from build123d import *

# Parameters (mm, degrees)
CROQUIS1_W              = 991
CROQUIS1_H              = 1639
SALIENTE_EXTRUIR1_DEPTH = 5
CROQUIS2_W              = 971
CROQUIS2_H              = 1619
CORTAR_EXTRUIR1_DEPTH   = 2
CROQUIS3_W              = 991
CROQUIS3_H              = 1639
CROQUIS3_W_2            = 989
CROQUIS3_H_2            = 1637
SALIENTE_EXTRUIR2_DEPTH = 30
CROQUIS4_W              = 991
CROQUIS4_H              = 1639
CROQUIS4_W_2            = 921
CROQUIS4_H_2            = 1569
SALIENTE_EXTRUIR3_DEPTH = 1
CROQUIS5_R              = 2.5
CORTAR_EXTRUIR2_DEPTH   = 1


with BuildPart() as part:
    # Croquis1 → Saliente-Extruir1 (new body)
    with BuildSketch(Plane.XY):
        Rectangle(CROQUIS1_W, CROQUIS1_H)
    extrude(amount=SALIENTE_EXTRUIR1_DEPTH)

    # Croquis2 → Cortar-Extruir1 (cut)
    with BuildSketch(Plane.XY.offset(5)):
        Rectangle(CROQUIS2_W, CROQUIS2_H)
    extrude(amount=-CORTAR_EXTRUIR1_DEPTH, mode=Mode.SUBTRACT)

    # Croquis3 → Saliente-Extruir2 (add)
    with BuildSketch(Plane(origin=(0, 0, 0), x_dir=(-1, 0, 0), z_dir=(0, 0, -1))):
        Rectangle(CROQUIS3_W, CROQUIS3_H)
        Rectangle(CROQUIS3_W_2, CROQUIS3_H_2, mode=Mode.SUBTRACT)
    extrude(amount=SALIENTE_EXTRUIR2_DEPTH)

    # Croquis4 → Saliente-Extruir3 (add)
    with BuildSketch(Plane(origin=(0, 0, -30), x_dir=(-1, 0, 0), z_dir=(0, 0, -1))):
        Rectangle(CROQUIS4_W, CROQUIS4_H)
        Rectangle(CROQUIS4_W_2, CROQUIS4_H_2, mode=Mode.SUBTRACT)
    extrude(amount=-SALIENTE_EXTRUIR3_DEPTH)

    # Croquis5 → Cortar-Extruir2 (cut)
    with BuildSketch(Plane(origin=(0, 0, -30), x_dir=(-1, 0, 0), z_dir=(0, 0, -1))):
        with Locations((-478, 0)):
            Circle(CROQUIS5_R)
        with Locations((478, 0)):
            Circle(CROQUIS5_R)
        with BuildLine():
            Line((-473, 652.5), (-473, 648.5))
            ThreePointArc((-473, 648.5), (-478, 643.5), (-483, 648.5))
            Line((-483, 648.5), (-483, 652.5))
            ThreePointArc((-483, 652.5), (-478, 657.5), (-473, 652.5))
        make_face()
        with BuildLine():
            Line((-473, 398.5), (-473, 402.5))
            ThreePointArc((-473, 402.5), (-478, 407.5), (-483, 402.5))
            Line((-483, 402.5), (-483, 398.5))
            ThreePointArc((-483, 398.5), (-478, 393.5), (-473, 398.5))
        make_face()
        with BuildLine():
            Line((-473, -652.5), (-473, -648.5))
            ThreePointArc((-473, -648.5), (-478, -643.5), (-483, -648.5))
            Line((-483, -648.5), (-483, -652.5))
            ThreePointArc((-483, -652.5), (-478, -657.5), (-473, -652.5))
        make_face()
        with BuildLine():
            Line((-473, -398.5), (-473, -402.5))
            ThreePointArc((-473, -402.5), (-478, -407.5), (-483, -402.5))
            Line((-483, -402.5), (-483, -398.5))
            ThreePointArc((-483, -398.5), (-478, -393.5), (-473, -398.5))
        make_face()
        with BuildLine():
            Line((473, -652.5), (473, -648.5))
            ThreePointArc((473, -648.5), (478, -643.5), (483, -648.5))
            Line((483, -648.5), (483, -652.5))
            ThreePointArc((483, -652.5), (478, -657.5), (473, -652.5))
        make_face()
        with BuildLine():
            Line((473, -398.5), (473, -402.5))
            ThreePointArc((473, -402.5), (478, -407.5), (483, -402.5))
            Line((483, -402.5), (483, -398.5))
            ThreePointArc((483, -398.5), (478, -393.5), (473, -398.5))
        make_face()
        with BuildLine():
            Line((473, 398.5), (473, 402.5))
            ThreePointArc((473, 402.5), (478, 407.5), (483, 402.5))
            Line((483, 402.5), (483, 398.5))
            ThreePointArc((483, 398.5), (478, 393.5), (473, 398.5))
        make_face()
        with BuildLine():
            Line((473, 652.5), (473, 648.5))
            ThreePointArc((473, 648.5), (478, 643.5), (483, 648.5))
            Line((483, 648.5), (483, 652.5))
            ThreePointArc((483, 652.5), (478, 657.5), (473, 652.5))
        make_face()
    extrude(amount=-CORTAR_EXTRUIR2_DEPTH, mode=Mode.SUBTRACT)


solid = part.part
Work out the finished part from the listing and answer in its coordinate system (mm). A direction names the side the tool comes from. Round coordinates to 2 decimals unless told otherwise and drop trailing zeros. Write each loop counter-clockwise with the first axis right and the second up, starting at its lowest first coordinate (ties: lowest second). Pieces come first, ordered by that corner, then holes. Notation, with made-up numbers: M 84,88.5 L 89,88.5 A20 ccw 89,106.5 Z; hole C 81,-5 d5. An arc over 180 degrees is marked long. Use a Markdown table: item, result.
1) Consider line 1 (Y direction, x = -478, z = -29.45); line 2 (X direction, y = 152, z = -6); line 3 (Y direction, x = 113.5, z = -12). Determine where each line is inside the solid, lowest interval first. Write a range as [from, to].
Taken from the geometry:
| item | result |
|---|---|
| line 1 | y = [-819.5, -657.5], [-643.5, -407.5], [-393.5, -2.5], [2.5, 393.5], [407.5, 643.5], [657.5, 819.5] |
| line 2 | x = [-495.5, -494.5], [494.5, 495.5] |
| line 3 | y = [-819.5, -818.5], [818.5, 819.5] |
2) The part is cut by section B-B on x = 169. Give the vertices of the cut face in (y, z).
Taken from the geometry:
| item | result |
|---|---|
| outline | M -819.5,-30 L -784.5,-30 L -784.5,-29 L -818.5,-29 L -818.5,0 L 818.5,0 L 818.5,-29 L 784.5,-29 L 784.5,-30 L 819.5,-30 L 819.5,5 L 809.5,5 L 809.5,3 L -809.5,3 L -809.5,5 L -819.5,5 Z |
3) Determine the mould class of faces 1 (the face through (495.5, -11, -12)), 2 (the face through (-7, 11, 3)), 3 (the face through (494.5, -11, -14)) for opening direction Z: pulls with the +Z half, pulls with the -Z half, needs draft (parallel to the pull), parting line crosses it, or undercut.
Taken from the geometry:
| item | result |
|---|---|
| face 1 | needs draft |
| face 2 | pulls with the +Z half |
| face 3 | undercut |
4) The part is cut by section C-C on y = 135.5. Give the vertices of the cut face in (x, z).
Taken from the geometry:
| item | result |
|---|---|
| outline | M -495.5,-30 L -460.5,-30 L -460.5,-29 L -494.5,-29 L -494.5,0 L 494.5,0 L 494.5,-29 L 460.5,-29 L 460.5,-30 L 495.5,-30 L 495.5,5 L 485.5,5 L 485.5,3 L -485.5,3 L -485.5,5 L -495.5,5 Z |
5) The part is cut by section A-A on z = -18. Give the vertices of the cut face in (x, y).
Taken from the geometry:
| item | result |
|---|---|
| outline | M -495.5,-819.5 L 495.5,-819.5 L 495.5,819.5 L -495.5,819.5 Z; hole M -494.5,-818.5 L 494.5,-818.5 L 494.5,818.5 L -494.5,818.5 Z |
6) Flat-ended cylindrical pins translate along their axes: pin 1 (4 mm diameter, centred on x = -478, y = 0, fed in from -Z); pin 2 (5 mm diameter, centred on x = -130.5, y = 356, fed in from +Z). Find the tip coordinate at first contact, or state that the pin passes through.
Taken from the geometry:
| item | result |
|---|---|
| pin 1 | stops at z = 0 |
| pin 2 | stops at z = 3 |
7) Which of the six approach directions +Z, -Z, +X, -X, +Y, -Y give full straight-line access (tool end or side, diameter ignored) to faces 4 (the face through (-495.5, -11, -12)), 5 (the face through (-494.5, -11, -14))?
Taken from the geometry:
| item | result |
|---|---|
| face 4 | +Z, -Z, -X, +Y, -Y |
| face 5 | none |
